Could you check a few things on this drawing? It's one solid part, dimensions in mm from its lowest x, y, z. A direction names the side the tool comes from. Coordinates: 2 decimals unless noted, no trailing zeros. Order: outer loops, then holes, each group sorted by start corner. A loop starts at its lowest first (then second) coordinate and runs counter-clockwise, first axis right, second up. Notation, with made-up numbers: (69.25, -36) -> (111.25, -36) arc R26 cw to (111.25, -15) -> close; hole circle Ø11 at (41.25, 51). An arc over 180 degrees is marked (long way). Answer as CSV lines item,"result".
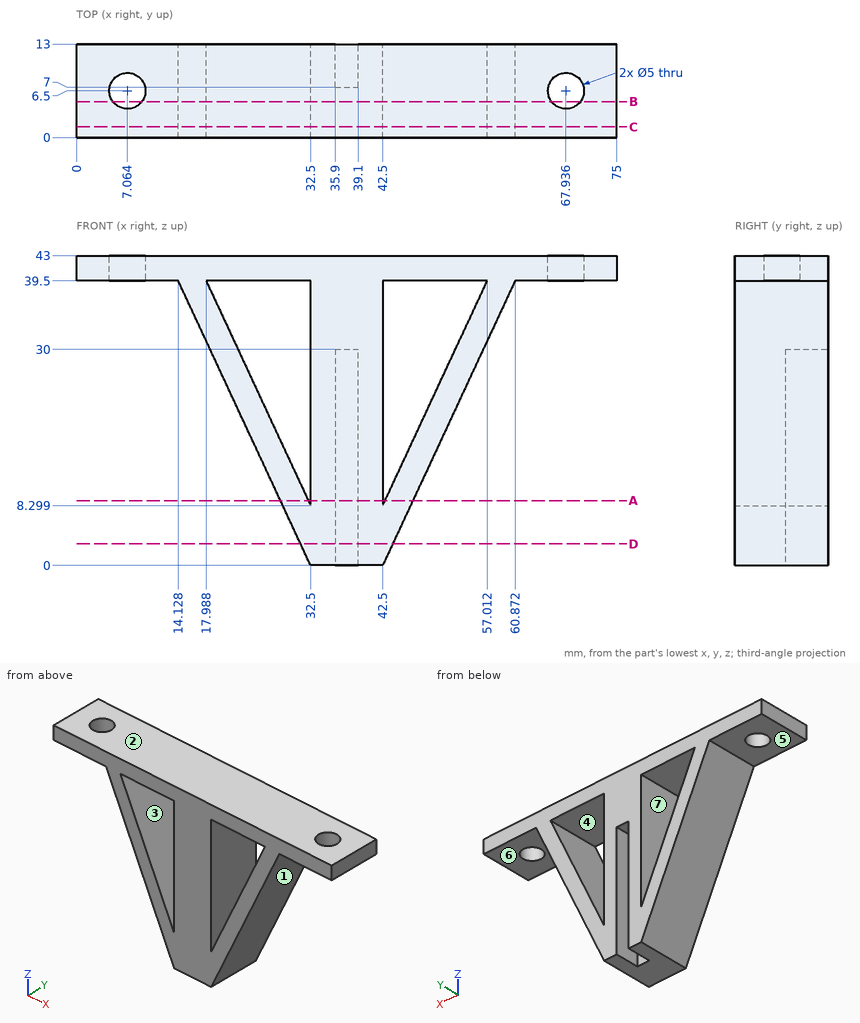
Q1. We'd pull the mould along X, two halves only. Please class the marked faces 1, 2, 3 and 4: pulls with the +X half, pulls with the -X half, needs draft (parallel to the pull), parting line crosses it, or undercut.
Solution:
face 1,"pulls with the +X half"
face 2,"needs draft"
face 3,"undercut"
face 4,"undercut"
Q2. Imagine slicing it at C-C (y = 1.5). List the corners of the cut face in (x, z) for me.
Solution:
outline,"(0, 39.5) -> (14.13, 39.5) -> (32.5, 0) -> (42.5, 0) -> (60.87, 39.5) -> (75, 39.5) -> (75, 43) -> (0, 43) -> close; hole (17.99, 39.5) -> (32.5, 8.3) -> (32.5, 39.5) -> close; hole (42.5, 8.3) -> (57.01, 39.5) -> (42.5, 39.5) -> close"
Q3. Imagine slicing it at B-B (y = 5). List the corners of the cut face in (x, z) for me.
Solution:
outline,"(0, 39.5) -> (5.06, 39.5) -> (5.06, 43) -> (0, 43) -> close; (9.06, 39.5) -> (14.13, 39.5) -> (32.5, 0) -> (42.5, 0) -> (60.87, 39.5) -> (65.94, 39.5) -> (65.94, 43) -> (9.06, 43) -> close; (69.94, 39.5) -> (75, 39.5) -> (75, 43) -> (69.94, 43) -> close; hole (17.99, 39.5) -> (32.5, 8.3) -> (32.5, 39.5) -> close; hole (42.5, 8.3) -> (57.01, 39.5) -> (42.5, 39.5) -> close"
Q4. For P1, Ø5, axis at y = 10.5, z = 19, coming from the +X side; P2, Ø3, axis at y = 10.5, z = 21, coming from the -X side (3 decimals); P3, Ø1.5, axis at y = 9, z = 15.5, coming from the +X side, each with a flat end and sliding along its axis, tell me the tip position at first contact or that it passes through.
Solution:
P1,"x = 52.5"
P2,"x = 22.035"
P3,"x = 50.06"
Q5. If I drill on line 1 (X direction, y = 9.75, z = 35.5); line 2 (X direction, y = 9.25, z = 36.5); line 3 (Z direction, x = 66, y = 2.75), over which ranges is the centre line in solid material (lowest first)?
Solution:
line 1,"15.99 to 19.85, 32.5 to 42.5, 55.15 to 59.01"
line 2,"15.52 to 19.38, 32.5 to 42.5, 55.62 to 59.48"
line 3,"39.5 to 43"
Q6. Imagine slicing it at D-D (z = 3). List the corners of the cut face in (x, y) for me.
Solution:
outline,"(31.1, 0) -> (43.9, 0) -> (43.9, 13) -> (39.1, 13) -> (39.1, 7) -> (35.9, 7) -> (35.9, 13) -> (31.1, 13) -> close"
Q7. Which directions (+Z, -Z, +X, -X, +Y, -Y) give clear straight access to the entire face, cutting with the end or side of a thin tool? Please do the marked faces 5, 6 and 7.
Solution:
face 5,"-Z, -X, +Y, -Y"
face 6,"-Z, +X, +Y, -Y"
face 7,"+Y, -Y"
Q8. Imagine slicing it at A-A (z = 9). List the corners of the cut face in (x, y) for me.
Solution:
outline,"(28.31, 0) -> (32.17, 0) -> (32.17, 13) -> (28.31, 13) -> close; (32.5, 0) -> (42.5, 0) -> (42.5, 13) -> (39.1, 13) -> (39.1, 7) -> (35.9, 7) -> (35.9, 13) -> (32.5, 13) -> close; (42.83, 0) -> (46.69, 0) -> (46.69, 13) -> (42.83, 13) -> close"
